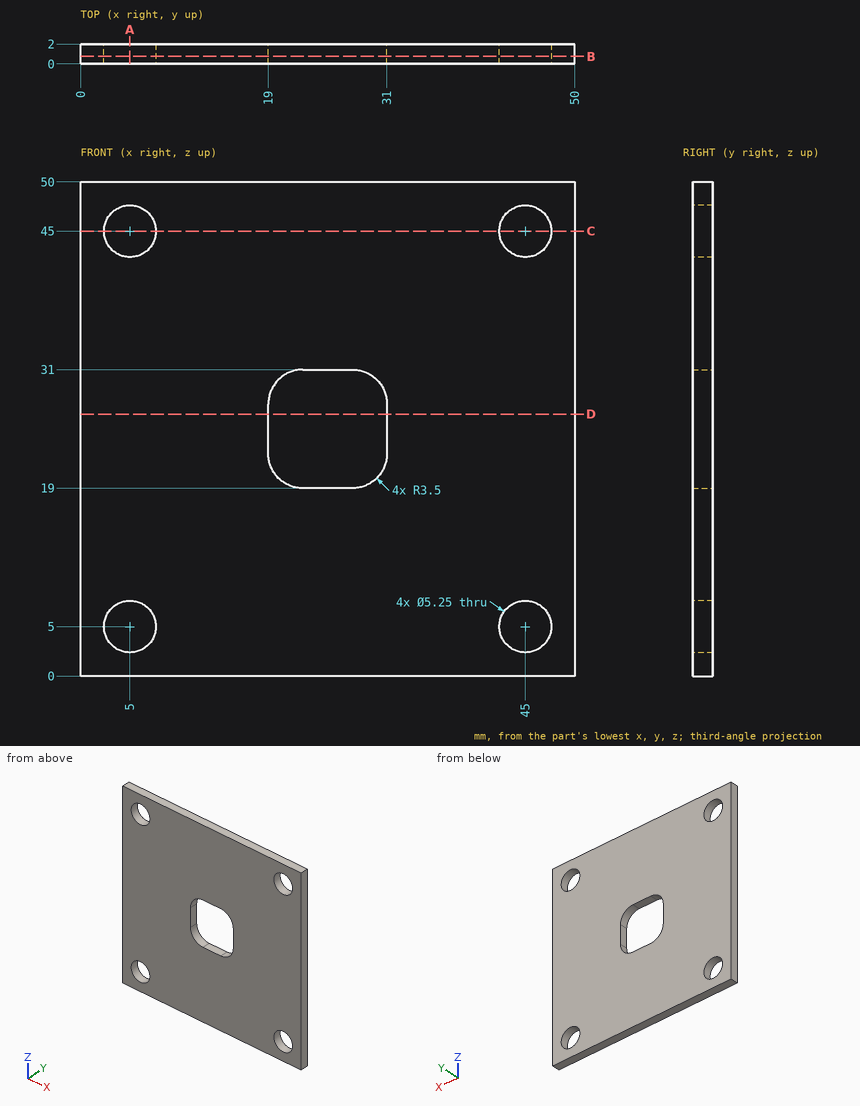
Could you check a few things on this drawing? It's one solid part, dimensions in mm from its lowest x, y, z. Give positions to 0.01 mm unless a question says otherwise; leave off trailing zeros. Order: outer loops, then holes, each group sorted by start corner. A loop starts at its lowest first (then second) coordinate and runs counter-clockwise, first axis right, second up.
1. Suppose I cut it at B-B (y = 0.75). Write out the boundary of the cut face in (x, z) (3 decimals), plus the area to 3 significant figures.
Answers below:
outline: (0, 0) - (50, 0) - (50, 50) - (0, 50) - close; hole circle Ø5.25 at (5, 5); hole circle Ø5.25 at (5, 45); hole (19, 22.5) arc R3.5 ccw to (22.5, 19) - (27.5, 19) arc R3.5 ccw to (31, 22.5) - (31, 27.5) arc R3.5 ccw to (27.5, 31) - (22.5, 31) arc R3.5 ccw to (19, 27.5) - close; hole circle Ø5.25 at (45, 5); hole circle Ø5.25 at (45, 45)
area: 2,280 mm2
2. Suppose I cut it at C-C (z = 45). Write out the boundary of the cut face in (x, y) (3 decimals), plus the area to 3 significant figures.
Answers below:
outline: (0, 0) - (2.375, 0) - (2.375, 2) - (0, 2) - close; (7.625, 0) - (42.375, 0) - (42.375, 2) - (7.625, 2) - close; (47.625, 0) - (50, 0) - (50, 2) - (47.625, 2) - close
area: 79.0 mm2
3. Suppose I cut it at A-A (x = 5). Write out the boundary of the cut face in (y, z) (3 decimals), plus the area to 3 significant figures.
Answers below:
outline: (0, 0) - (2, 0) - (2, 2.375) - (0, 2.375) - close; (0, 7.625) - (2, 7.625) - (2, 42.375) - (0, 42.375) - close; (0, 47.625) - (2, 47.625) - (2, 50) - (0, 50) - close
area: 79.0 mm2
4. Suppose I cut it at D-D (z = 26.5). Write out the boundary of the cut face in (x, y).
Answers below:
outline: (0, 0) - (19, 0) - (19, 2) - (0, 2) - close; (31, 0) - (50, 0) - (50, 2) - (31, 2) - close
5. I need wall thicknesses on L1, parallel to Z at x = 5, y = 1.4 (3 decimals); L2, parallel to Z at x = 26.5, y = 0.3; L3, parallel to X at y = 0.95, z = 46. Which ranges of each line are inside material? Lowest first, please.
Answers below:
L1: z = 0 to 2.375, 7.625 to 42.375, 47.625 to 50
L2: z = 0 to 19, 31 to 50
L3: x = 0 to 2.57, 7.43 to 42.57, 47.43 to 50
6. For pin 1 (3 mm diameter, centred on x = 45, z = 5, fed in from -Y) (1 decimal), with a flat end and sliding along its axis, tell me the tip position at first contact or that it passes through.
Answers below:
pin 1: passes through
